Can you work these out from the drawing? Everything is in mm from the part's minimum corner. A direction names the side the tool comes from. Round coordinates to 2 decimals unless told otherwise and drop trailing zeros. Order: outer loops, then holes, each group sorted by start corner. A loop starts at its lowest first (then second) coordinate and runs counter-clockwise, first axis right, second up. Notation, with made-up numbers: (36.25, 72.25) -> (64.25, 72.25) arc R24 cw to (64.25, 84.25) -> close; hole circle Ø5 at (-6.5, 40.5). An arc over 180 degrees is marked (long way). One line per item, written item: value.
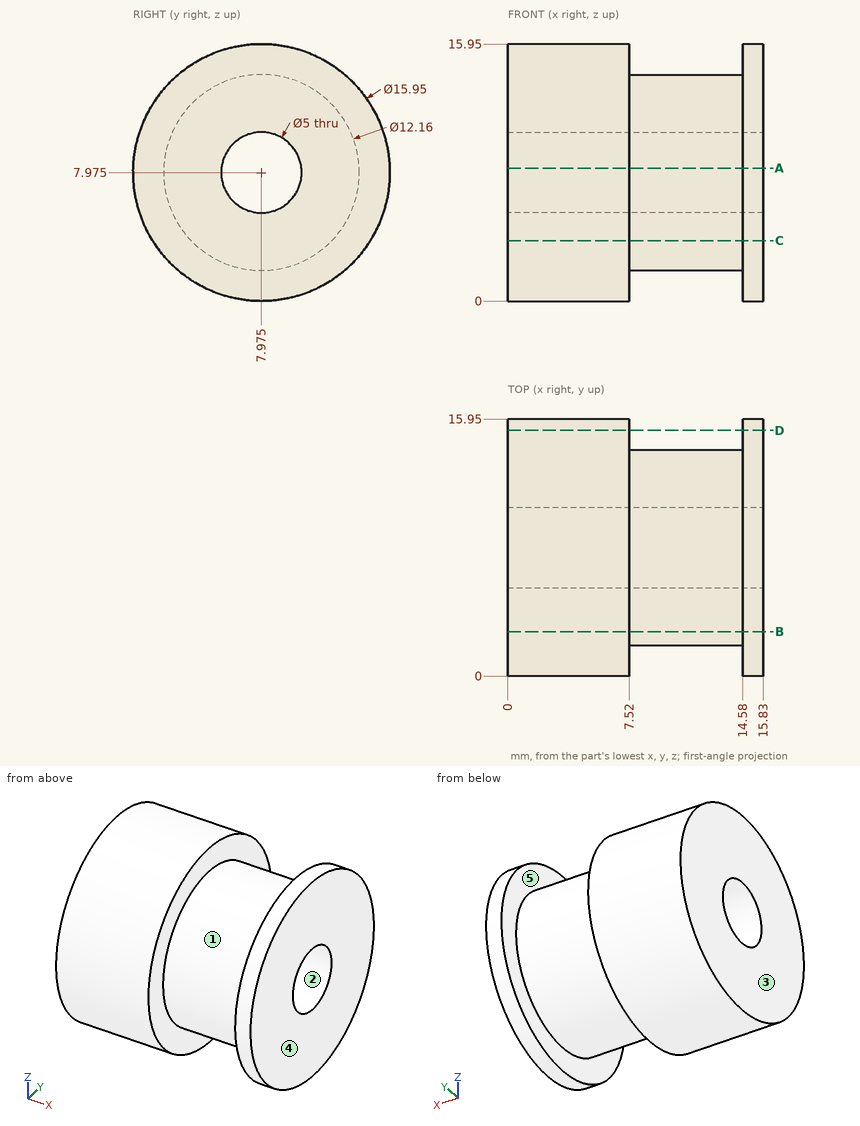
Q1. I want a section at D-D on y = 15.25. Write out the boundary of the cut face in (x, z), then the cut area to 3 significant figures.
Answers:
outline: (0, 4.71) -> (7.52, 4.71) -> (7.52, 11.24) -> (0, 11.24) -> close; (14.58, 4.71) -> (15.83, 4.71) -> (15.83, 11.24) -> (14.58, 11.24) -> close
area: 57.3 mm2
Q2. I need wall thicknesses on line 1 along X through (y, z) = (4, 14.5); line 2 along Y through (x, z) = (3.5, 8); line 3 along Y through (x, z) = (2.25, 10.25). Which ranges of each line are inside material? Lowest first, please.
Answers:
line 1: 0 to 7.52, 14.58 to 15.83
line 2: 0 to 5.48, 10.47 to 15.95
line 3: 0.33 to 6.94, 9.01 to 15.62
Q3. Which directions (+Z, -Z, +X, -X, +Y, -Y) give clear straight access to the entire face, cutting with the end or side of a thin tool? Please do the marked faces 4 and 5.
Answers:
face 4: +Z, -Z, +X, +Y, -Y
face 5: none
Q4. If we mould it in two halves opening along Y, with no side actions, what happens to the marked faces 1, 2 and 3? For each: pulls with the +Y half, pulls with the -Y half, needs draft (parallel to the pull), parting line crosses it, or undercut.
Answers:
face 1: parting line crosses it
face 2: undercut
face 3: needs draft
Q5. I want a section at A-A on z = 8.25. Write out the boundary of the cut face in (x, y).
Answers:
outline: (0, 0) -> (7.52, 0) -> (7.52, 1.9) -> (14.58, 1.9) -> (14.58, 0) -> (15.83, 0) -> (15.83, 5.49) -> (0, 5.49) -> close; (0, 10.46) -> (15.83, 10.46) -> (15.83, 15.95) -> (14.58, 15.95) -> (14.58, 14.05) -> (7.52, 14.05) -> (7.52, 15.95) -> (0, 15.95) -> close
Q6. I want a section at B-B on y = 2.75. Write out the boundary of the cut face in (x, z).
Answers:
outline: (0, 1.95) -> (7.52, 1.95) -> (7.52, 4.87) -> (14.58, 4.87) -> (14.58, 1.95) -> (15.83, 1.95) -> (15.83, 14) -> (14.58, 14) -> (14.58, 11.08) -> (7.52, 11.08) -> (7.52, 14) -> (0, 14) -> close
Q7. For P1, Ø8, axis at x = 8, z = 3, coming from the -Y side; P2, Ø4.5, axis at y = 7.975, z = 7.975, coming from the +X side; P3, Ø2, axis at x = 10.5, z = 9, coming from the +Y side, each with a flat end and sliding along its axis, tell me the tip position at first contact or that it passes through.
Answers:
P1: y = 0.06
P2: through
P3: y = 14.05
Q8. I want a section at C-C on z = 3.75. Write out the boundary of the cut face in (x, y).
Answers:
outline: (0, 1.21) -> (7.52, 1.21) -> (7.52, 3.6) -> (14.58, 3.6) -> (14.58, 1.21) -> (15.83, 1.21) -> (15.83, 14.74) -> (14.58, 14.74) -> (14.58, 12.35) -> (7.52, 12.35) -> (7.52, 14.74) -> (0, 14.74) -> close
